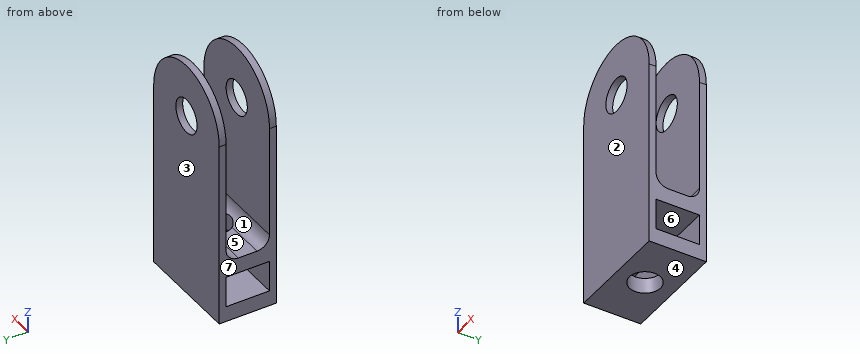
Autodesk Inventor part; units mm, degrees
ref_plane "Plan de construction1" through (0, 8.1, 0) normal (0, 1, 0) x (1, 0, 0)
ref_plane "Plan de construction2" through (0, 4.6, 0) normal (0, -1, 0) x (1, 0, 0)
ref_plane "YZ Plane" through (0, 0, 0) normal (1, 0, 0) x (0, 1, 0)
sketch "Esquisse1" plane through (0, 0, 0) normal (0, 1, 0) x (-1, 0, 0)
  circle A0 centre (0, 0) radius 8.5
  circle A1 centre (0, 0) radius 2.75
  line L0 (0, 0) -> (0, -30)
  line L1 (8.5, -30) -> (8.5, 0)
  line L2 (-8.5, -30) -> (-8.5, 0)
  line L3 (8.5, -30) -> (-8.5, -30)
  dimension "d0" = 17
  dimension "d1" = 5.5
  dimension "d4" = 30
  dimension "d5" = 30
  dimension "d6" = 30
extrude "Extrusion1" add sketch "Esquisse1" along normal blind 1.1
ref_plane "Plan de construction1" through (0, 8.1, 0) normal (0, 1, 0) x (1, 0, 0)
sketch "Esquisse3" plane through (0, 8.1, 0) normal (0, 1, 0) x (1, 0, 0)
  arc A0 (-8.5, 0) -> (8.5, 0) centre (0, 0) ccw
  line L0 (-8.5, 20) -> (-8.5, 0)
  line L1 (8.5, 0) -> (8.5, 20)
  line L2 (-8.5, 30) -> (-8.5, 15)
  line L3 (8.5, 30) -> (-8.5, 30)
  line L4 (8.5, 15) -> (8.5, 30)
  circle A1 centre (0, 0) radius 2.75
extrude "Extrusion3" add sketch "Esquisse3" along normal blind 1.1
ref_plane "Plan de construction2" through (0, 4.6, 0) normal (0, -1, 0) x (1, 0, 0)
sketch "Esquisse7" plane through (0, 4.6, 0) normal (0, -1, 0) x (1, 0, 0)
  line L0 (8.5, -30) -> (-8.5, -30)
  line L1 (-8.5, -30) -> (8.5, -30)
  line L2 (8.5, -30) -> (8.5, -20)
  line L3 (8.5, -20) -> (-8.5, -20)
  line L4 (-8.5, -20) -> (-8.5, -30)
  point P0 (0, 0)
  dimension "d41" = 10
extrude "Extrusion5" add sketch "Esquisse7" along normal mid plane 7
sketch "Esquisse8" plane through (8.5, 0, 0) normal (1, 0, 0) x (0, 0, -1)
  line L0 (20, 8.1) -> (0, 8.1)
  line L1 (30, 0) -> (30, 9.2)
  line L2 (0, 0) -> (30, 0)
  line L3 (25, 8.1) -> (27.5, 8.1)
  line L4 (27.5, 8.1) -> (22.5, 8.1)
  line L5 (22.5, 8.1) -> (22.5, 1.1)
  line L6 (22.5, 1.1) -> (27.5, 1.1)
  line L7 (27.5, 1.1) -> (27.5, 8.1)
  line L8 (0, 9.2) -> (30, 9.2)
  dimension "d43" = 5
  dimension "d44" = 7
  dimension "d45" = 1.1
  dimension "d46" = 2.5
extrude "Extrusion6" cut sketch "Esquisse8" against normal through all
sketch "Esquisse9" plane through (8.5, 0, -30) normal (0, 0, -1) x (-1, 0, 0)
  line L0 (5.75, 9.2) -> (11.25, 9.2)
  line L1 (8.5, 9.2) -> (8.5, 0)
  point P0 (8.5, 4.6)
hole "Perçage3" at (0, 4.6, -30) direction (0, 0, 1) diameter 5 end through all
fillet "Congé3" radius 2 2 edges at (0, 8.1, -20) (0, 1.1, -20)
properties part number "bielle sup"
Input: part model. Units: mm. Frame: model coordinates. Face numbers are marked on the shaded views. A direction names the side the tool comes from. Give positions to 0.01 mm unless a question says otherwise; leave off trailing zeros. Order: outer loops, then holes, each group sorted by start corner. A loop starts at its lowest first (then second) coordinate and runs counter-clockwise, first axis right, second up. Notation, with made-up numbers: (-7.5, 17) - (16.5, 17) arc R7 ccw to (16.5, 25) - close; hole circle Ø7 at (-4, -7.5). An arc over 180 degrees is marked (long way). Answer as a JSON object with one key per item and string values. Group by question number.
Q1. Cut plane A-A, the plane y = 4.6. Output: boundary loops of the cut face in (x, z), then the cut area to 3 significant figures.
Q2. First-contact query: pin 1 Ø1 at (y, z) = (2.5, -3.5) entering from -X; pin 2 Ø1.5 at (x, y) = (-5, 4) entering from +Z; pin 3 Ø1.5 at (x, y) = (-2.5, 1) entering from +Z; pin 4 Ø4 at (x, y) = (3, 4.5) entering from +Z. Flat tips, straight axial feed; report the tip coordinate or a pass-through.
Q3. Cut plane C-C, the plane x = 0. Output: boundary loops of the cut face in (y, z).
Q4. Mould query, pull axis Y, two halves, no side actions, for the marked faces 1, 2, 3 and 4. Classes: pulls with the +Y half, pulls with the -Y half, needs draft (parallel to the pull), parting line crosses it, or undercut.
Q5. Line query: probe 1 along Y at (x, z) = (-4, -14); probe 2 along X at (y, z) = (8.75, 0); probe 3 along Z at (x, y) = (6.75, 3.5). Output: solid intervals per line, ascending.
Q6. Cut plane B-B, the plane z = -23.5. Output: boundary loops of the cut face in (x, y).
Q7. Cut plane D-D, the plane x = -7.5. Output: boundary loops of the cut face in (y, z), then the cut area to 3 significant figures.
Q8. Set-up query: the marked faces 5, 6 and 7. Return all of +Z, -Z, +X, -X, +Y, -Y with unobstructed straight access to the full face (end or side cutting, diameter ignored); none if empty.
Results:
{
 "1": {"outline": "(-8.5, -30) - (-2.5, -30) - (-2.5, -27.5) - (-8.5, -27.5) - close; (-8.5, -22.5) - (-2.5, -22.5) - (-2.5, -20) - (-8.5, -20) - close; (2.5, -30) - (8.5, -30) - (8.5, -27.5) - (2.5, -27.5) - close; (2.5, -22.5) - (8.5, -22.5) - (8.5, -20) - (2.5, -20) - close", "area": "60.0 mm^2"},
 "2": {"pin 1": "through", "pin 2": "z = -20", "pin 3": "z = 8.32", "pin 4": "z = -19.91"},
 "3": {"outline": "(0, -30) - (2.1, -30) - (2.1, -27.5) - (1.1, -27.5) - (1.1, -22.5) - (2.1, -22.5) - (2.1, -19.73) arc R2 cw to (1.1, -18) - (1.1, -2.75) - (0, -2.75) - close; (0, 2.75) - (1.1, 2.75) - (1.1, 8.5) - (0, 8.5) - close; (7.1, -30) - (9.2, -30) - (9.2, -2.75) - (8.1, -2.75) - (8.1, -18) arc R2 cw to (7.1, -19.73) - (7.1, -22.5) - (8.1, -22.5) - (8.1, -27.5) - (7.1, -27.5) - close; (8.1, 2.75) - (9.2, 2.75) - (9.2, 8.5) - (8.1, 8.5) - close"},
 "4": {"face 1": "undercut", "face 2": "pulls with the -Y half", "face 3": "pulls with the +Y half", "face 4": "needs draft"},
 "5": {"probe 1": "0 to 1.1, 8.1 to 9.2", "probe 2": "-8.5 to -2.75, 2.75 to 8.5", "probe 3": "-30 to -27.5, -22.5 to -20"},
 "6": {"outline": "(-8.5, 0) - (8.5, 0) - (8.5, 1.1) - (-8.5, 1.1) - close; (-8.5, 8.1) - (8.5, 8.1) - (8.5, 9.2) - (-8.5, 9.2) - close"},
 "7": {"outline": "(0, -30) - (9.2, -30) - (9.2, 4) - (8.1, 4) - (8.1, -18) arc R2 cw to (6.1, -20) - (3.1, -20) arc R2 cw to (1.1, -18) - (1.1, 4) - (0, 4) - close; hole (1.1, -27.5) - (8.1, -27.5) - (8.1, -22.5) - (1.1, -22.5) - close", "area": "112 mm^2"},
 "8": {"face 5": "+Z, +X, -X", "face 6": "+X, -X", "face 7": "+Z, -Z, -X, +Y, -Y"}
}
